Verification items for this drawing (mm, ordinates from the low corner). Give positions to 0.01 mm unless a question says otherwise; leave off trailing zeros. Order: outer loops, then holes, each group sorted by start corner. A loop starts at its lowest first (then second) coordinate and runs counter-clockwise, first axis right, second up. Notation, with made-up numbers: M 3,20.5 L 60,20.5 A23 cw 60,54.5 Z; hole C -30,-15.75 d11. An arc over 180 degrees is marked long. One line per question, with ' | ' between items. Start each with the question number.
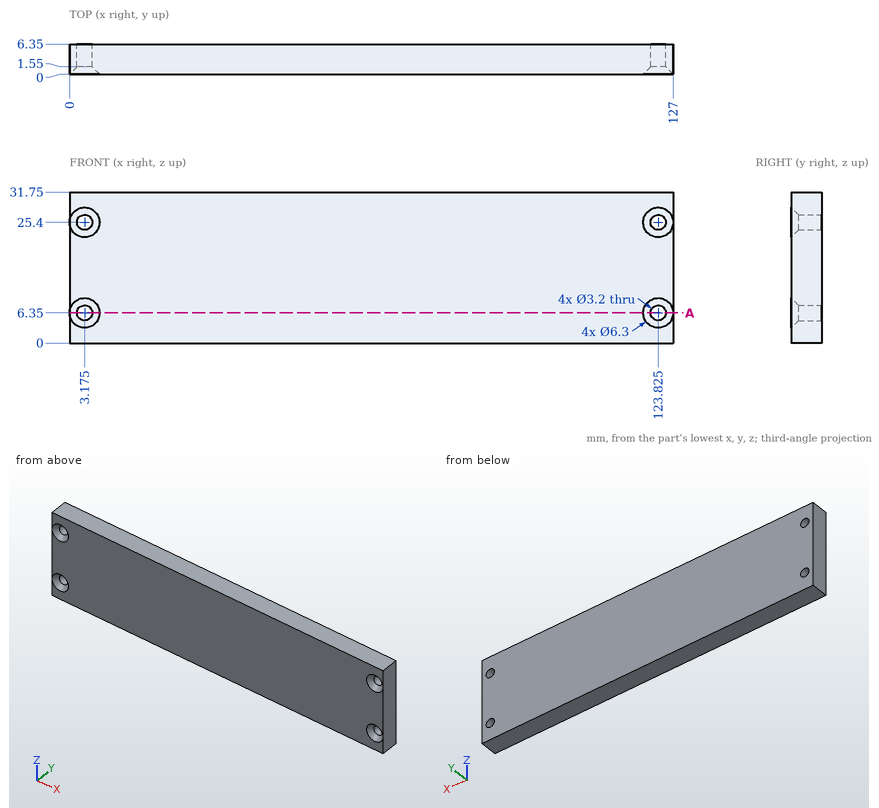
Item 1: Depth check by flat-ended pin: pin 1 (3.5 mm diameter, centred on x = 3.175, z = 6.35, fed in from -Y). Enter the tip coordinate at first touch or a pass-through.
Item 2: Cross-section at A-A, the plane z = 6.35. Record the cut outline in (x, y) (3 decimals), plus the area to 3 significant figures.
Item 3: Material ranges on line 1 along X through (y, z) = (5.4, 6.35) (3 decimals); line 2 along X through (y, z) = (3, 5.5), recorded low to high.
Outcome:
1) pin 1: stops at y = 1.4
2) outline: M 0,0 L 0.025,0 L 1.575,1.55 L 1.575,6.35 L 0,6.35 Z; M 4.775,1.55 L 6.325,0 L 120.675,0 L 122.225,1.55 L 122.225,6.35 L 4.775,6.35 Z; M 125.425,1.55 L 126.975,0 L 127,0 L 127,6.35 L 125.425,6.35 Z | area: 761 mm²
3) line 1: x = 0 to 1.575, 4.775 to 122.225, 125.425 to 127 | line 2: x = 0 to 1.82, 4.53 to 122.47, 125.18 to 127
